The model under review builds one solid part; all positions refer to its coordinate system, in mm. Face numbers are marked on the shaded views. A direction names the side the tool comes from. Round coordinates to 2 decimals unless told otherwise and drop trailing zeros. Order: outer loops, then holes, each group sorted by start corner. A loop starts at its lowest first (then second) coordinate and runs counter-clockwise, first axis right, second up. Notation, with made-up numbers: (62, 5) -> (92, 5) arc R25 ccw to (92, 34) -> close; hole circle Ø5 at (8, 65). An arc over 180 degrees is marked (long way). Use a Markdown table: item, result. Add a question column.
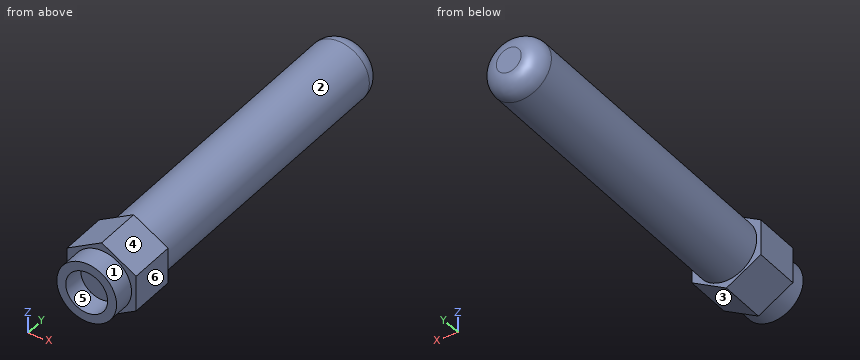
```python
from build123d import *

# Parameters (mm, degrees)
SKETCH1_R           = 3.81
SKETCH1_R_2         = 2.667
BOSS_EXTRUDE1_DEPTH = 2.794
BOSS_EXTRUDE2_DEPTH = 5.969
SKETCH4_R           = 3.8735
BOSS_EXTRUDE3_DEPTH = 40.64
FILLET1_R           = 2.286


with BuildPart() as part:
    # Sketch1 → Boss-Extrude1 (new body)
    with BuildSketch(Plane(origin=(0, 0, 0), x_dir=(1, 0, 0), z_dir=(0, 1, 0))):
        Circle(SKETCH1_R)
        Circle(SKETCH1_R_2, mode=Mode.SUBTRACT)
    extrude(amount=BOSS_EXTRUDE1_DEPTH)

    # Sketch3 → Boss-Extrude2 (add)
    with BuildSketch(Plane(origin=(0, 2.794, 0), x_dir=(1, 0, 0), z_dir=(0, 1, 0))):
        Polygon((-4.399409051, -2.286), (-4.399409051, 2.286), (0, 4.826), (4.399409051, 2.286), (4.399409051, -2.286), (0, -4.826), align=None)
    extrude(amount=BOSS_EXTRUDE2_DEPTH)

    # Sketch4 → Boss-Extrude3 (add)
    with BuildSketch(Plane(origin=(0, 8.763, 0), x_dir=(1, 0, 0), z_dir=(0, 1, 0))):
        Circle(SKETCH4_R)
    extrude(amount=BOSS_EXTRUDE3_DEPTH)

    # Fillet1
    fillet1_edges = [part.edges().sort_by_distance(p)[0] for p in [
        (-3.8735, 49.403, 0),
    ]]
    fillet(fillet1_edges, radius=FILLET1_R)


solid = part.part
```
Q1. Machinability: for the marked faces 1, 2 and 3, which of the approach directions +Z, -Z, +X, -X, +Y, -Y give a long, thin tool a straight path to every point of the face, cutting with its end or side? Answer none if there is none.
Q2. Insertion check: pin 1 (5 mm diameter, centred on y = 37, z = 0.5, fed in from -X); pin 2 (3 mm diameter, centred on y = 16.5, z = 3, fed in from +X); pin 3 (2 mm diameter, centred on y = 13, z = 3.5, fed in from -X). Each pin has a flat end and moves straight along its axis. Give the tip position at first contact, or say it passes through.
Q3. Wall thickness on line 1 (Z direction, x = 0, y = 2.2); line 2 (Y direction, x = 0, z = 1.5): over which ranges is each line inside the solid? List them lowest first. Write a range as [from, to].
Q4. Mouldability with a two-part tool opening along Z and no side actions: class the marked faces 4, 5 and 6 as pulls with the +Z half, pulls with the -Z half, needs draft (parallel to the pull), parting line crosses it, or undercut.
Q5. Add section A-A (y = 11.5). Write out the cut boundary in (x, z), then the cut area to 3 significant figures.
Report:
| question | item | result |
|---|---|---|
| 1 | face 1 | -Y |
| 1 | face 2 | +Y |
| 1 | face 3 | -Z, +X, +Y, -Y |
| 2 | pin 1 | stops at x = -3.87 |
| 2 | pin 2 | stops at x = 3.57 |
| 2 | pin 3 | stops at x = -2.96 |
| 3 | line 1 | z = [-3.81, -2.67], [2.67, 3.81] |
| 3 | line 2 | y = [2.79, 49.4] |
| 4 | face 4 | pulls with the +Z half |
| 4 | face 5 | undercut |
| 4 | face 6 | needs draft |
| 5 | outline | circle Ø7.75 at (0, 0) |
| 5 | area | 47.1 mm² |
